Print and shaded views of the part. All mm, measured from the part's lowest x, y and z. Give positions to 0.01 mm unless a question says otherwise; leave off trailing zeros. Write each loop counter-clockwise with the first axis right and the second up, starting at its lowest first coordinate (ties: lowest second). Pieces come first, ordered by that corner, then holes. Notation, with made-up numbers: (-26, -4) -> (-20, -4) arc R18 ccw to (-20, 31) -> close; hole circle Ø10 at (24.25, -40). An arc over 180 degrees is marked (long way). Put each result on its own line as item: value.
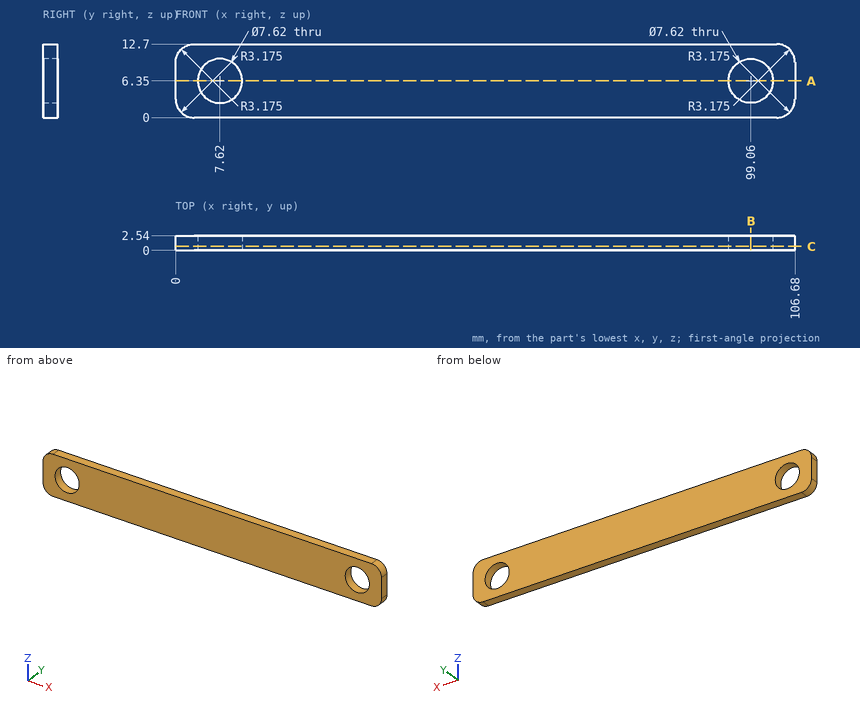
1) Slice it at B-B (x = 99.06). Write the cut outline in (y, z).
Filled sheet:
outline: (0, 0) -> (2.54, 0) -> (2.54, 2.54) -> (0, 2.54) -> close; (0, 10.16) -> (2.54, 10.16) -> (2.54, 12.7) -> (0, 12.7) -> close
2) Wall check: L1, parallel to X at y = 0.5, z = 6.35; L2, parallel to Z at x = 7.62, y = 0.85; L3, parallel to X at y = 2.25, z = 3. Give the ranges that are in metal, low to high.
Filled sheet:
L1: 0 to 3.81, 11.43 to 95.25, 102.87 to 106.68
L2: 0 to 2.54, 10.16 to 12.7
L3: 0 to 5.81, 9.43 to 97.25, 100.87 to 106.68
3) Slice it at A-A (z = 6.35). Write the cut outline in (x, y).
Filled sheet:
outline: (0, 0) -> (3.81, 0) -> (3.81, 2.54) -> (0, 2.54) -> close; (11.43, 0) -> (95.25, 0) -> (95.25, 2.54) -> (11.43, 2.54) -> close; (102.87, 0) -> (106.68, 0) -> (106.68, 2.54) -> (102.87, 2.54) -> close
4) Pin check, flat tips, straight feed: pin 1 (4 mm diameter, centred on x = 82.5, z = 8, fed in from -Y); pin 2 (4.5 mm diameter, centred on x = 7.62, z = 6.35, fed in from +Y). Stop position of each tip, or through.
Filled sheet:
pin 1: y = 0
pin 2: through
5) Slice it at C-C (y = 0.7). Write the cut outline in (x, z) (3 decimals).
Filled sheet:
outline: (0, 3.175) arc R3.175 ccw to (3.175, 0) -> (103.505, 0) arc R3.175 ccw to (106.68, 3.175) -> (106.68, 9.525) arc R3.175 ccw to (103.505, 12.7) -> (3.175, 12.7) arc R3.175 ccw to (0, 9.525) -> close; hole circle Ø7.62 at (7.62, 6.35); hole circle Ø7.62 at (99.06, 6.35)
